For this review, use the dimensioned drawing (mm, ordinates from the lowest corner) and the shaded views. Round coordinates to 2 decimals unless told otherwise and drop trailing zeros. Write each loop counter-clockwise with the first axis right and the second up, starting at its lowest first coordinate (ties: lowest second). Pieces come first, ordered by that corner, then holes. Notation, with made-up numbers: (-24, 66.25) -> (-6, 66.25) arc R13 ccw to (-6, 77.25) -> close; hole circle Ø6 at (-22, 87). An arc over 180 degrees is marked (long way). Write each question's results on one line, items separated by ' | '. Start each with the question number.
Item 1: Add section B-B (y = 14.1). State the section outline as (x, z) points, plus the area to 4 significant figures.
Item 2: To check wall thickness, follow line 1 along Y through (x, z) = (1.5, 0.9); line 2 along Y through (x, z) = (14.75, 2.2). State the ranges of each line that lie inside material, in increasing order.
Item 3: Add section A-A (x = 15.2). State the section outline as (y, z) points.
Item 4: Clearance check with a flat-ended pin moving along its axis: pin 1 (1.1 mm diameter, centred on x = 8.1, y = 14.1, fed in from +Z). State where the tip first meets the part, or that it passes through.
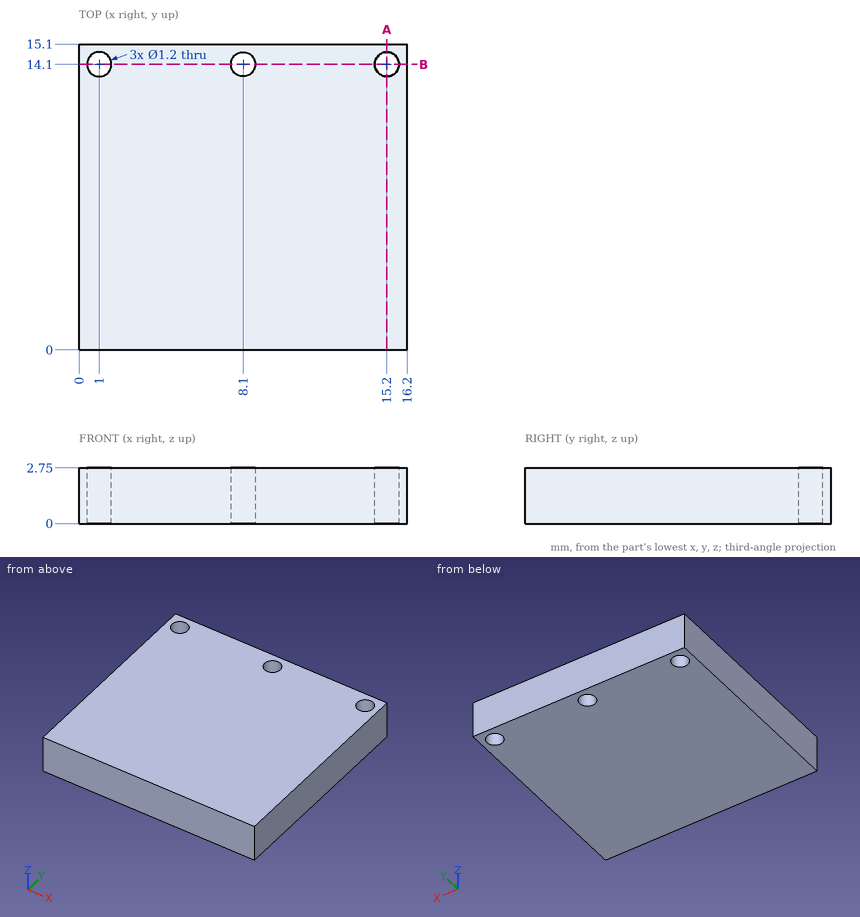
Responses:
1) outline: (0, 0) -> (0.4, 0) -> (0.4, 2.75) -> (0, 2.75) -> close; (1.6, 0) -> (7.5, 0) -> (7.5, 2.75) -> (1.6, 2.75) -> close; (8.7, 0) -> (14.6, 0) -> (14.6, 2.75) -> (8.7, 2.75) -> close; (15.8, 0) -> (16.2, 0) -> (16.2, 2.75) -> (15.8, 2.75) -> close | area: 34.65 mm^2
2) line 1: y = 0 to 13.77, 14.43 to 15.1 | line 2: y = 0 to 13.7, 14.5 to 15.1
3) outline: (0, 0) -> (13.5, 0) -> (13.5, 2.75) -> (0, 2.75) -> close; (14.7, 0) -> (15.1, 0) -> (15.1, 2.75) -> (14.7, 2.75) -> close
4) pin 1: passes through
